Can you work these out from the model? Positions are in its coordinate system, mm. A direction names the side the tool comes from. Round coordinates to 2 decimals unless told otherwise and drop trailing zeros. Loops run counter-clockwise (first coordinate to the right, second up) from the corner with the lowest first, then second, coordinate; pieces in that order, holes last. Notation, with made-up numbers: (33, 40) -> (69, 40) arc R26 cw to (69, 71) -> close; hole circle Ø7 at (74, -19.5). An arc over 180 degrees is marked (long way). Write each question's results on one line, items separated by ' | '.
from build123d import *

# Parameters (mm, degrees)
SKETCH1_R           = 4.6
SKETCH1_R_2         = 3
BOSS_EXTRUDE1_DEPTH = 5.9
CHAMFER1_SIZE       = 0.15
CHAMFER2_SIZE       = 0.15
SKETCH2_R           = 4.6
BOSS_EXTRUDE2_DEPTH = 2.5
BOSS_EXTRUDE2_DRAFT = -37.234833982
SKETCH3_R           = 3
CUT_EXTRUDE1_DEPTH  = 2.5
SKETCH4_R           = 6.5
SKETCH4_R_2         = 3
BOSS_EXTRUDE3_DEPTH = 4
SKETCH5_R           = 5.5
SKETCH5_R_2         = 3
BOSS_EXTRUDE4_DEPTH = 5.5
CUT_EXTRUDE2_START  = -1.25
SKETCH6_R           = 6.5
SKETCH6_R_2         = 6
CUT_EXTRUDE2_DEPTH  = 1.25
BOSS_EXTRUDE5_START = -1.25
SKETCH7_R           = 6
SKETCH7_R_2         = 5.5
BOSS_EXTRUDE5_DEPTH = 1.25
FILLET1_R           = 0.25
SKETCH8_R           = 4.5
CUT_EXTRUDE3_DEPTH  = 4
CHAMFER4_SIZE       = 0.15
CHAMFER5_SIZE       = 0.15


with BuildPart() as part:
    # Sketch1 → Boss-Extrude1 (new body)
    with BuildSketch(Plane(origin=(0, 1, 0), x_dir=(-1, 0, 0), z_dir=(0, -1, 0))):
        with Locations(Location((-12.350088109, 22.338562584, 0), (0, 0, 90))):
            Circle(SKETCH1_R)
        with Locations(Location((-12.350088109, 22.338562584, 0), (0, 0, 90))):
            Circle(SKETCH1_R_2, mode=Mode.SUBTRACT)
    extrude(amount=BOSS_EXTRUDE1_DEPTH)

    # Chamfer1
    chamfer1_edges = [part.edges().sort_by_distance(p)[0] for p in [
        (12.350088109, 1, -17.738562584),
    ]]
    chamfer(chamfer1_edges, length=CHAMFER1_SIZE)

    # Chamfer2
    chamfer2_edges = [part.edges().sort_by_distance(p)[0] for p in [
        (12.350088109, 1, -19.338562584),
    ]]
    chamfer(chamfer2_edges, length=CHAMFER2_SIZE)


with BuildPart() as boss_extrude2_tool:
    # Sketch2 → Boss-Extrude2 (with draft: the straight prism first)
    with BuildSketch(Plane(origin=(0, -4.9, 0), x_dir=(-1, 0, 0), z_dir=(0, -1, 0))):
        with Locations(Location((-12.350088109, 22.338562584, 0), (0, 0, 90))):
            Circle(SKETCH2_R)
    extrude(amount=BOSS_EXTRUDE2_DEPTH)
    # Boss-Extrude2: the draft: its side faces are tilted about the plane it starts from
    boss_extrude2_sides = [boss_extrude2_tool.faces().sort_by_distance(p)[0] for p in [
        (12.350088109, -6.15, -17.738562584),
    ]]
    draft(boss_extrude2_sides, Plane(origin=(0, -4.9, 0), x_dir=(-1, 0, 0), z_dir=(0, -1, 0)), BOSS_EXTRUDE2_DRAFT)


with BuildPart() as part_1:
    add(part.part)

    # Boss-Extrude2: add boss_extrude2_tool
    add(boss_extrude2_tool.part)

    # Sketch3 → Cut-Extrude1 (cut)
    with BuildSketch(Plane(origin=(0, -4.9, 0), x_dir=(1, 0, 0), z_dir=(0, 1, 0))):
        with Locations(Location((12.350088109, 22.338562584, 0), (0, 0, 270))):
            Circle(SKETCH3_R)
    extrude(amount=-CUT_EXTRUDE1_DEPTH, mode=Mode.SUBTRACT)

    # Sketch4 → Boss-Extrude3 (add)
    with BuildSketch(Plane(origin=(0, -7.4, 0), x_dir=(-1, 0, 0), z_dir=(0, -1, 0))):
        with Locations(Location((-12.350088109, 22.338562584, 0), (0, 0, 90))):
            Circle(SKETCH4_R)
        with Locations(Location((-12.350088109, 22.338562584, 0), (0, 0, 270))):
            Circle(SKETCH4_R_2, mode=Mode.SUBTRACT)
    extrude(amount=BOSS_EXTRUDE3_DEPTH)

    # Sketch5 → Boss-Extrude4 (add)
    with BuildSketch(Plane.XZ.offset(11.4)):
        with Locations(Location((12.350088109, -22.338562584, 0), (0, 0, 270))):
            Circle(SKETCH5_R)
        with Locations(Location((12.350088109, -22.338562584, 0), (0, 0, 90))):
            Circle(SKETCH5_R_2, mode=Mode.SUBTRACT)
    extrude(amount=BOSS_EXTRUDE4_DEPTH)

    # Sketch6 → Cut-Extrude2 (cut)
    with BuildSketch(Plane.XZ.offset(11.4).offset(CUT_EXTRUDE2_START)):
        with Locations(Location((12.350088109, -22.338562584, 0), (0, 0, 270))):
            Circle(SKETCH6_R)
        with Locations(Location((12.350088109, -22.338562584, 0), (0, 0, 270))):
            Circle(SKETCH6_R_2, mode=Mode.SUBTRACT)
    extrude(amount=CUT_EXTRUDE2_DEPTH, mode=Mode.SUBTRACT)

    # Sketch7 → Boss-Extrude5 (add)
    with BuildSketch(Plane(origin=(0, -16.9, 0), x_dir=(-1, 0, 0), z_dir=(0, -1, 0)).offset(BOSS_EXTRUDE5_START)):
        with Locations(Location((-12.350088109, 22.338562584, 0), (0, 0, 90))):
            Circle(SKETCH7_R)
        with Locations(Location((-12.350088109, 22.338562584, 0), (0, 0, 90))):
            Circle(SKETCH7_R_2, mode=Mode.SUBTRACT)
    extrude(amount=BOSS_EXTRUDE5_DEPTH)

    # Fillet1
    fillet1_edges = [part_1.edges().sort_by_distance(p)[0] for p in [
        (12.350088109, -16.9, -16.338562584),
    ]]
    fillet(fillet1_edges, radius=FILLET1_R)

    # Sketch8 → Cut-Extrude3 (cut)
    with BuildSketch(Plane(origin=(0, -16.9, 0), x_dir=(-1, 0, 0), z_dir=(0, -1, 0))):
        with Locations(Location((-12.350088109, 22.338562584, 0), (0, 0, 90))):
            Circle(SKETCH8_R)
    extrude(amount=-CUT_EXTRUDE3_DEPTH, mode=Mode.SUBTRACT)

    # Chamfer4
    chamfer4_edges = [part_1.edges().sort_by_distance(p)[0] for p in [
        (12.350088109, -16.9, -17.838562584),
    ]]
    chamfer(chamfer4_edges, length=CHAMFER4_SIZE)

    # Chamfer5
    chamfer5_edges = [part_1.edges().sort_by_distance(p)[0] for p in [
        (12.350088109, -12.9, -25.338562584),
    ]]
    chamfer(chamfer5_edges, length=CHAMFER5_SIZE)


solid = part_1.part
1. We'd pull the mould along Z, two halves only. Please class faces 6 (the face through (12.592, -13.495, -16.844)), 7 (the face through (11, -15.65, -28)), 8 (the face through (11, -12.9, -19)): pulls with the +Z half, pulls with the -Z half, needs draft (parallel to the pull), parting line crosses it, or undercut.
Final values:
face 6: parting line crosses it | face 7: needs draft | face 8: undercut
2. On a 3-axis mill with a long thin cutter (end or side, diameter ignored), from which of +Z, -Z, +X, -X, +Y, -Y can I reach the whole of each face in a straight line? I mean faces 1 (the face through (7, -10.15, -19)), 2 (the face through (11, 1, -19)), 3 (the face through (11, -11.4, -28)), 4 (the face through (14.3, -8.76, -28.54)), 5 (the face through (10.59, -1.98, -26.59)). Say none if no direction works.
Final values:
face 1: -Y | face 2: +Z, -Z, +X, -X, +Y | face 3: none | face 4: +Y, -Y | face 5: +Y
3. Will these pins go through, and if not, where does the flat tip stop? pin 1 (1.5 mm diameter, centred on y = -9, z = -22.5, fed in from -X); pin 2 (3.5 mm diameter, centred on x = 12.35, z = -22.34, fed in from +Y); pin 3 (2 mm diameter, centred on y = -6.5, z = -18.5, fed in from -X); pin 4 (4 mm diameter, centred on x = 11, z = -21, fed in from -Y).
Final values:
pin 1: x = 5.85 | pin 2: through | pin 3: x = 6.8 | pin 4: y = -12.9
4. Please list where these lines run through material, in increasing order: line 1 (X direction, y = -14.25, z = -22.5); line 2 (Z direction, x = 12.5, y = -14); line 3 (X direction, y = -8.75, z = -22.5). Write a range as from..to.
Final values:
line 1: 6.85..7.85, 16.85..17.85 | line 2: -27.84..-26.84, -17.84..-16.84 | line 3: 5.85..9.35, 15.35..18.85
5. If we section it at A-A (y = -9.25): List the corners of the cut face in (x, z) for me, then the cut area to 3 significant figures.
Final values:
outline: circle Ø13 at (12.35, -22.34); hole circle Ø6 at (12.35, -22.34) | area: 104 mm2
6. If we section it at B-B (y = 0): List the corners of the cut face in (x, z) for me.
Final values:
outline: circle Ø9.2 at (12.35, -22.34); hole circle Ø6 at (12.35, -22.34)
